Check sheet for the modelled part. Datum: model origin and axes. Units: mm. Face numbers are marked on the shaded views. A direction names the side the tool comes from. Round coordinates to 2 decimals unless told otherwise and drop trailing zeros. Write each loop counter-clockwise with the first axis right and the second up, starting at its lowest first coordinate (ties: lowest second). Pieces come first, ordered by that corner, then holes. Notation, with made-up numbers: (-12, 58.25) -> (31, 58.25) arc R16 cw to (31, 88.25) -> close; hole circle Ø3 at (-18.75, 25). An arc over 180 degrees is marked (long way). Answer as a JSON object with one key per item and string values. Group by question number.
```python
from build123d import *

# Parameters (mm, degrees)
F1_DEPTH = 25.4
F2_R     = 6.35
F3_DEPTH = 25.4
F5_DEPTH = 25.4


with BuildPart() as f1:
    # F0 (on Front) → F1 (new body)
    with BuildSketch(Plane.XZ):
        Polygon((0, 31.75), (0, 0), (69.85, 0), (69.85, 12.7), (25.4, 12.7), (25.4, 31.75), align=None)
    extrude(amount=F1_DEPTH)

    # F2 (on face) → F3 (cut)
    with BuildSketch(Plane.XZ.offset(25.4)):
        with BuildLine():
            ThreePointArc((0, 19.05), (12.7, 31.182884), (25.4, 19.05))
            Line((25.4, 19.05), (25.4, 31.75))
            Line((25.4, 31.75), (0, 31.75))
            Line((0, 31.75), (0, 19.05))
        make_face()
        with Locations((12.7, 19.05)):
            Circle(F2_R)
    extrude(amount=-F3_DEPTH, mode=Mode.SUBTRACT)

    # F4 (on face) → F5 (cut)
    with BuildSketch(Plane.XY.offset(12.7)):
        with BuildLine():
            ThreePointArc((38.1, -19.05), (42.590128, -17.190128), (44.45, -12.7))
            ThreePointArc((44.45, -12.7), (42.590128, -8.209872), (38.1, -6.35))
            ThreePointArc((38.1, -6.35), (31.75, -12.7), (38.1, -19.05))
        make_face()
        with BuildLine():
            ThreePointArc((38.1, -6.35), (42.590128, -8.209872), (44.45, -12.7))
            ThreePointArc((44.45, -12.7), (42.590128, -17.190128), (38.1, -19.05))
            Line((38.1, -19.05), (57.15, -19.05))
            ThreePointArc((57.15, -19.05), (50.8, -12.7), (57.15, -6.35))
            Line((57.15, -6.35), (38.1, -6.35))
        make_face()
        with BuildLine():
            ThreePointArc((63.5, -12.7), (61.640128, -8.209872), (57.15, -6.35))
            ThreePointArc((57.15, -6.35), (50.8, -12.7), (57.15, -19.05))
            ThreePointArc((57.15, -19.05), (61.640128, -17.190128), (63.5, -12.7))
        make_face()
        with BuildLine():
            ThreePointArc((57.15, 0), (69.088758, -12.7), (57.15, -25.4))
            Line((57.15, -25.4), (69.85, -25.4))
            Line((69.85, -25.4), (69.85, 0))
            Line((69.85, 0), (57.15, 0))
        make_face()
    extrude(amount=-F5_DEPTH, mode=Mode.SUBTRACT)


solid = f1.part
```
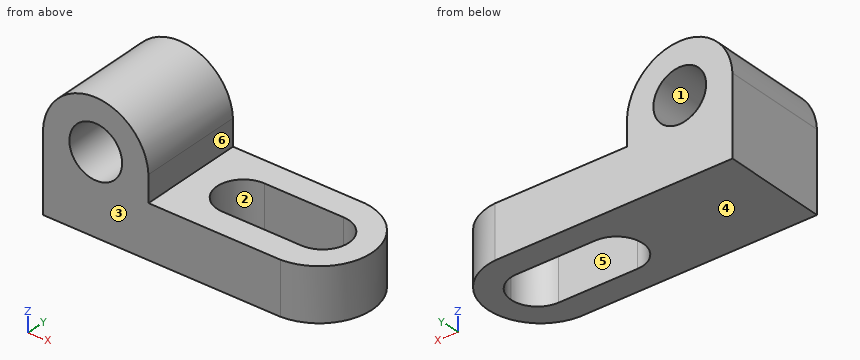
(1) Scan lines: line 1 along Z through (x, y) = (12.7, -7); line 2 along Z through (x, y) = (34, -3.75); line 3 along X through (y, z) = (-15.75, 9.5). Record each from-to range of solid material in increasing order.
(2) Section check A-A on y = -10. Record the cut outline in (x, z).
(3) Go/stop test with flat-tipped pins: pin 1 Ø4 at (y, z) = (-16, 25.5) entering from -X; pin 2 Ø5 at (x, z) = (61, 14.5) entering from -Y; pin 3 Ø7 at (y, z) = (-8.5, 16) entering from +X. Record where each tip stops, or that it passes through.
(4) Section check D-D on z = 9.5. Record the cut outline in (x, y), then the cut area to 3 significant figures.
(5) Section check C-C on x = 12.7. Record the cut outline in (y, z).
(6) Release check for a two-part mould opening along Y. For the marked faces 1, 2 and 3 record: pulls with the +Y half, pulls with the -Y half, needs draft (parallel to the pull), parting line crosses it, or undercut.
(7) Section check B-B on z = 17. Record the cut outline in (x, y), then the cut area to 3 significant figures.
(8) Access from +Z, -Z, +X, -X, +Y, -Y to the whole of each face (thin tool, end or side, straight path). Record for the marked faces 4, 5 and 6.
Data:
{
 "1": {"line 1": "z = 0 to 12.7, 25.4 to 31.18", "line 2": "z = 0 to 12.7", "line 3": "x = 0 to 32.53, 62.72 to 68.72"},
 "2": {"outline": "(0, 0) -> (32.35, 0) -> (32.35, 12.7) -> (25.4, 12.7) -> (25.4, 19.05) arc R12.71 ccw to (0, 19.05) -> close; (62.9, 0) -> (68.8, 0) -> (68.8, 12.7) -> (62.9, 12.7) -> close; hole circle Ø12.7 at (12.7, 19.05)"},
 "3": {"pin 1": "stops at x = 1.02", "pin 2": "stops at y = -25.09", "pin 3": "stops at x = 68.72"},
 "4": {"outline": "(0, -25.4) -> (57.15, -25.4) arc R12.72 ccw to (57.15, 0) -> (0, 0) -> close; hole (38.1, -19.05) -> (57.15, -19.05) arc R6.35 ccw to (57.15, -6.35) -> (38.1, -6.35) arc R6.35 ccw to start", "area": "1,320 mm²"},
 "5": {"outline": "(-25.4, 0) -> (0, 0) -> (0, 12.7) -> (-25.4, 12.7) -> close; (-25.4, 25.4) -> (0, 25.4) -> (0, 31.18) -> (-25.4, 31.18) -> close"},
 "6": {"face 1": "needs draft", "face 2": "undercut", "face 3": "pulls with the -Y half"},
 "7": {"outline": "(0, -25.4) -> (6.69, -25.4) -> (6.69, 0) -> (0, 0) -> close; (18.71, -25.4) -> (25.4, -25.4) -> (25.4, 0) -> (18.71, 0) -> close", "area": "340 mm²"},
 "8": {"face 4": "-Z, +X, -X, +Y, -Y", "face 5": "+Z, -Z", "face 6": "+Z, +X, +Y, -Y"}
}
